from build123d import *

# Parameters (mm, degrees)
F0_R     = 11.05
F1_DEPTH = 7


with BuildPart() as f1:
    # F0 (on Top) → F1 (new body)
    with BuildSketch(Plane.XY):
        with BuildLine():
            Line((18.114797, 18.648818), (13.55, 26.842903))
            ThreePointArc((13.55, 26.842903), (0, 40.392903), (-13.55, 26.842903))
            Line((-13.55, 26.842903), (-18.163027, 18.52472))
            ThreePointArc((-18.163027, 18.52472), (-15.631693, 9.690215), (-24.466198, 7.15888))
            Line((-24.466198, 7.15888), (-29.039817, -1.088241))
            ThreePointArc((-29.039817, -1.088241), (-34.68947, -20.455852), (-14.823439, -23.972062))
            Line((-14.823439, -23.972062), (-6.713385, -23.972062))
            ThreePointArc((-6.713385, -23.972062), (0, -17.258678), (6.713385, -23.972062))
            Line((6.713385, -23.972062), (14.823439, -23.972062))
            ThreePointArc((14.823439, -23.972062), (34.661194, -20.501168), (29.135954, -1.134821))
            Line((29.135954, -1.134821), (24.568158, 7.064647))
            ThreePointArc((24.568158, 7.064647), (15.549392, 9.630052), (18.114797, 18.648818))
        make_face()
        with Locations((-23.179692, -13.305501)):
            Circle(F0_R, mode=Mode.SUBTRACT)
        with Locations((23.179692, -13.305501)):
            Circle(F0_R, mode=Mode.SUBTRACT)
        Circle(F0_R, mode=Mode.SUBTRACT)
        with Locations((0, 26.842903)):
            Circle(F0_R, mode=Mode.SUBTRACT)
    extrude(amount=F1_DEPTH)


solid = f1.part
Geometry: final body of the model. Coordinates: model frame, mm. A direction names the side the tool comes from. Coordinates: 2 decimals unless noted, no trailing zeros. Order: outer loops, then holes, each group sorted by start corner. A loop starts at its lowest first (then second) coordinate and runs counter-clockwise, first axis right, second up.
1) Set-up query: faces 1 (the flat face through (-11, -23.972, 3)), 2 (the cylindrical face through (0.3, 40.39, 3.45)). Return all of +Z, -Z, +X, -X, +Y, -Y with unobstructed straight access to the full face (end or side cutting, diameter ignored); none if empty.
Result sheet:
face 1: +Z, -Z, -Y
face 2: +Z, -Z, +Y
2) Section C-C (z = 1.75). Return loops of the section in (x, y).
Result sheet:
outline: (-29.04, -1.09) arc R13.55 ccw (long way) to (-14.82, -23.97) - (-6.71, -23.97) arc R6.71 cw to (6.71, -23.97) - (14.82, -23.97) arc R13.55 ccw (long way) to (29.14, -1.13) - (24.57, 7.06) arc R6.63 cw to (18.11, 18.65) - (13.55, 26.84) arc R13.55 ccw to (-13.55, 26.84) - (-18.16, 18.52) arc R6.5 cw to (-24.47, 7.16) - close; hole circle Ø22.1 at (-23.18, -13.31); hole circle Ø22.1 at (0, 0); hole circle Ø22.1 at (0, 26.84); hole circle Ø22.1 at (23.18, -13.31)
3) Section A-A (x = 0). Return loops of the section in (y, z).
Result sheet:
outline: (-17.26, 0) - (-11.05, 0) - (-11.05, 7) - (-17.26, 7) - close; (11.05, 0) - (15.79, 0) - (15.79, 7) - (11.05, 7) - close; (37.89, 0) - (40.39, 0) - (40.39, 7) - (37.89, 7) - close
4) Draft query along Y for faces 3 (the cylindrical face through (29.12, -3.99, 3.45)), 4 (the cylindrical face through (34.49, -20.77, 3.45)), 5 (the cylindrical face through (-15.56, 9.82, 3.45)), 6 (the flat face through (-15.824, 22.742, 3.451)). Return one class per face: released by +Y, released by -Y, zero draft, split by the parting line, or undercut.
Result sheet:
face 3: undercut
face 4: split by the parting line
face 5: undercut
face 6: released by +Y
5) Ray query, probe 1 along Y at (x, z) = (0, 2.25); probe 2 along X at (y, z) = (-18, 5); probe 3 along X at (y, z) = (-16, 4.5). Return the intervals inside material, ascending.
Result sheet:
probe 1: y = -17.26 to -11.05, 11.05 to 15.79, 37.89 to 40.39
probe 2: x = -35.89 to -33.18, -13.18 to -3.07, 3.07 to 13.18, 33.18 to 35.89
probe 3: x = -36.46 to -33.9, -12.46 to 12.46, 33.9 to 36.46
6) First-contact query: P1, Ø1.5, axis at y = 23.5, z = 2, coming from the +X side; P2, Ø3.5, axis at x = -12.5, z = 5, coming from the -Y side; P3, Ø1.5, axis at x = -1, z = 1, coming from the -Y side; P4, Ø1.5, axis at x = -8, y = 18, coming from the -Z side. Flat tips, straight axial feed; report the tip coordinate or a pass-through.
Result sheet:
P1: stops at x = 15.83
P2: stops at y = -23.97
P3: stops at y = -17.49
P4: stops at z = 0
7) Section B-B (y = 30). Return loops of the section in (x, z).
Result sheet:
outline: (-13.18, 0) - (-10.59, 0) - (-10.59, 7) - (-13.18, 7) - close; (10.59, 0) - (13.18, 0) - (13.18, 7) - (10.59, 7) - close
8) Section D-D (x = -19). Return loops of the section in (y, z).
Result sheet:
outline: (-26.19, 0) - (-23.53, 0) - (-23.53, 7) - (-26.19, 7) - close; (-3.08, 0) - (6.77, 0) - (6.77, 7) - (-3.08, 7) - close
